Work out the finished part from the listing and answer in its coordinate system (mm). A direction names the side the tool comes from. Round coordinates to 2 decimals unless told otherwise and drop trailing zeros. Order: outer loops, then holes, each group sorted by start corner. A loop starts at its lowest first (then second) coordinate and runs counter-clockwise, first axis right, second up. Notation, with made-up numbers: M -27,84.5 L -2,84.5 A17 cw -2,107.5 Z; hole C 30.5,-13 d2. An arc over 180 degrees is marked long. Return JSON: item names as keys, results as strings.
from build123d import *

# Parameters (mm, degrees)
F1_DEPTH = 66.5611065924


# Not quite as in the source:
# - the program builds the solid bodies; features that only make, move or delete a surface that nothing else refers to are left out


with BuildPart() as f1:
    # F0 (on Front) → F1 (new body)
    with BuildSketch(Plane.XZ):
        Polygon((-28.4163840115, 12.6286381856), (-35.0520461798, -35.7411280274), (-14.6560901776, -35.7411280274), (0, -18.0393829942), (13.2530285046, -10.4401372373), (43.007966131, -10.4401372373), (43.007966131, 12.6286381856), (-11.0137574375, 12.6286381856), align=None)
    extrude(amount=-F1_DEPTH)


solid = f1.part
Item 1: Find section A-A (y = 35). Determine the outline of the cut face in (x, z).
Output:
{"outline": "M -35.05,-35.74 L -14.66,-35.74 L 0,-18.04 L 13.25,-10.44 L 43.01,-10.44 L 43.01,12.63 L -28.42,12.63 Z"}
Item 2: Consider line 1 along Z through (x, y) = (18.5, 8); line 2 along X through (y, z) = (39, -1.5); line 3 along Z through (x, y) = (6, 20). Determine where each line is inside the solid, lowest interval first. Write a range as [from, to].
Output:
{"line 1": "z = [-10.44, 12.63]", "line 2": "x = [-30.35, 43.01]", "line 3": "z = [-14.6, 12.63]"}
Item 3: Each of these flat-tipped pins is pushed along its axis until it touches: pin 1 (2 mm diameter, centred on x = -4, z = 5.5, fed in from -Y); pin 2 (1.5 mm diameter, centred on y = 23.5, z = -6.5, fed in from -X); pin 3 (2 mm diameter, centred on x = 22, y = 28.5, fed in from -Z); pin 4 (8 mm diameter, centred on x = 1, y = 40.5, fed in from -Z). Where does it stop, or does it pass through?
Output:
{"pin 1": "stops at y = 0", "pin 2": "stops at x = -31.14", "pin 3": "stops at z = -10.44", "pin 4": "stops at z = -21.66"}
Item 4: Find section C-C (z = -4.5). Determine the outline of the cut face in (x, y).
Output:
{"outline": "M -30.77,0 L 43.01,0 L 43.01,66.56 L -30.77,66.56 Z"}
Item 5: Which of the six approach directions +Z, -Z, +X, -X, +Y, -Y give full straight-line access (tool end or side, diameter ignored) to faces 1 (the flat face through (8, 33, 12.629)), 2 (the flat face through (28, 33, -10.44))?
Output:
{"face 1": "+Z, +X, -X, +Y, -Y", "face 2": "-Z, +X, +Y, -Y"}
Item 6: Find section B-B (x = 34.5). Determine the outline of the cut face in (y, z).
Output:
{"outline": "M 0,-10.44 L 66.56,-10.44 L 66.56,12.63 L 0,12.63 Z"}
